Here's how the part is built. I have some questions about the finished solid (model axes, mm). Face numbers are marked on the shaded views. A direction names the side the tool comes from. Give positions to 0.01 mm unless a question says otherwise; leave off trailing zeros. Loops run counter-clockwise (first coordinate to the right, second up) from the corner with the lowest first, then second, coordinate; pieces in that order, holes last. Notation, with made-up numbers: (55, 50.5) - (75, 50.5) arc R15 cw to (75, 77.5) - close; hole circle Ø7 at (73, 35.5). An arc over 180 degrees is marked (long way). Use one line per item in the form item = value.
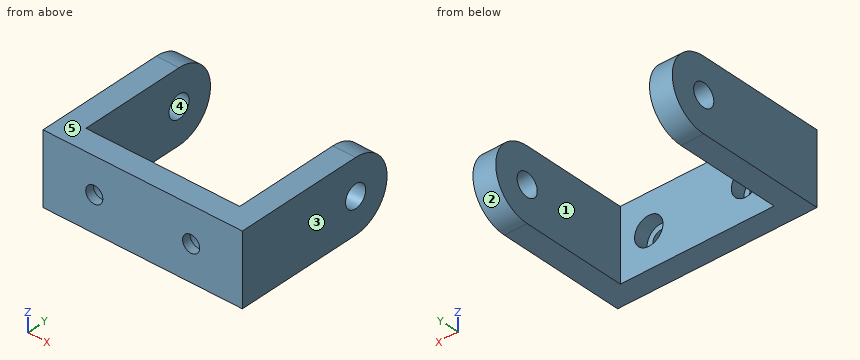
from build123d import *

# Parameters (mm, degrees)
SKETCH1_W           = 70
SKETCH1_H           = 25
BOSS_EXTRUDE1_DEPTH = 8
SKETCH2_R           = 3
CUT_EXTRUDE1_DEPTH  = 9
SKETCH2_3_R         = 5
CUT_EXTRUDE2_DEPTH  = 5
SKETCH3_R           = 4
BOSS_EXTRUDE2_DEPTH = 8


with BuildPart() as part:
    # Sketch1 → Boss-Extrude1 (new body)
    with BuildSketch(Plane(origin=(0, 0, 0), x_dir=(1, 0, 0), z_dir=(0, 1, 0))):
        with Locations((8.045977011, 1.83908046)):
            Rectangle(SKETCH1_W, SKETCH1_H)
    extrude(amount=BOSS_EXTRUDE1_DEPTH)

    # Sketch2 → Cut-Extrude1 (cut, through all)
    with BuildSketch(Plane(origin=(0, 8, 0), x_dir=(1, 0, 0), z_dir=(0, 1, 0))):
        with Locations((25.045977011, 1.83908046)):
            Circle(SKETCH2_R)
    cut_extrude1 = extrude(amount=-CUT_EXTRUDE1_DEPTH, mode=Mode.SUBTRACT)

    # Sketch2<3> → Cut-Extrude2 (cut)
    with BuildSketch(Plane(origin=(0, 8, 0), x_dir=(1, 0, 0), z_dir=(0, 1, 0))):
        with Locations((25.045977011, 1.83908046)):
            Circle(SKETCH2_3_R)
    cut_extrude2 = extrude(amount=-CUT_EXTRUDE2_DEPTH, mode=Mode.SUBTRACT)

    # Sketch3 → Boss-Extrude2 (add)
    with BuildSketch(Plane(origin=(43.045977011, 0, 0), x_dir=(0, 0, -1), z_dir=(1, 0, 0))):
        with BuildLine():
            Line((-10.66091954, 45), (-10.66091954, 8))
            Line((-10.66091954, 8), (14.33908046, 8))
            Line((14.33908046, 8), (14.33908046, 45))
            ThreePointArc((14.33908046, 45), (1.83908046, 57.5), (-10.66091954, 45))
        make_face()
        with Locations((1.83908046, 45)):
            Circle(SKETCH3_R, mode=Mode.SUBTRACT)
    boss_extrude2 = extrude(amount=-BOSS_EXTRUDE2_DEPTH)

    # Mirror1: Cut-Extrude1, Cut-Extrude2, Boss-Extrude2 across plane
    add(cut_extrude1.mirror(Plane(origin=(8.045977011, 0, 0), x_dir=(0, 0, 1), z_dir=(1, 0, 0))), mode=Mode.SUBTRACT)
    add(cut_extrude2.mirror(Plane(origin=(8.045977011, 0, 0), x_dir=(0, 0, 1), z_dir=(1, 0, 0))), mode=Mode.SUBTRACT)
    add(boss_extrude2.mirror(Plane(origin=(8.045977011, 0, 0), x_dir=(0, 0, 1), z_dir=(1, 0, 0))))


solid = part.part
(1) If we section it at A-A (y = 24.5): List the corners of the cut face in (x, z) for me.
Geometry says:
outline = (-26.95, -14.34) - (-18.95, -14.34) - (-18.95, 10.66) - (-26.95, 10.66) - close; (35.05, -14.34) - (43.05, -14.34) - (43.05, 10.66) - (35.05, 10.66) - close
(2) If we section it at C-C (x = -16): List the corners of the cut face in (y, z) for me, plus the area to 3 significant figures.
Geometry says:
outline = (0, -14.34) - (8, -14.34) - (8, 10.66) - (0, 10.66) - close
area = 200 mm²
(3) If we section it at D-D (z = -10.25): List the corners of the cut face in (x, y) for me, plus the area to 3 significant figures.
Geometry says:
outline = (-26.95, 0) - (43.05, 0) - (43.05, 54.25) - (35.05, 54.25) - (35.05, 8) - (-18.95, 8) - (-18.95, 54.25) - (-26.95, 54.25) - close
area = 1,300 mm²
(4) If we section it at B-B (z = -3): Give the number of separate pieces and of enclosed holes in the cut face, plus the area to 3 significant figures.
Geometry says:
separate_pieces = 5
enclosed_holes = 0
area = 1,100 mm²
(5) For the marked faces 1 and 2, which set-ups out of +Z, -Z, +X, -X, +Y, -Y let a thin tool reach every point of the face, with its end or its side?
Geometry says:
face_1 = +Z, -Z, +Y
face_2 = +X, -X, +Y
(6) Thinking about a two-plate mould opening in Z: for the marked faces 3, 4 and 5, which applies, pulls with the +Z half, pulls with the -Z half, needs draft (parallel to the pull), parting line crosses it, or undercut?
Geometry says:
face_3 = needs draft
face_4 = undercut
face_5 = pulls with the +Z half
(7) For P1, Ø9, axis at x = -8.95, z = -1.84, coming from the -Y side; P2, Ø11, axis at x = -11, z = -2, coming from the +Y side; P3, Ø5, axis at x = 23.5, z = -0.5, coming from the +Y side, each with a flat end and sliding along its axis, tell me the tip position at first contact or that it passes through.
Geometry says:
P1 = 0
P2 = 8
P3 = 3
(8) If I drill on probe 1 along X at (y, z) = (36, -9.5); probe 2 along Y at (x, z) = (39, -1.5); probe 3 along X at (y, z) = (7.5, -2.5), over which ranges is the centre line in solid material (lowest first)?
Geometry says:
probe_1 = -26.95 to -18.95, 35.05 to 43.05
probe_2 = 0 to 41.01, 48.99 to 57.5
probe_3 = -26.95 to -13.91, -4 to 20.09, 30 to 43.05
